from build123d import *

# Parameters (mm, degrees)
SKETCH1_W           = 39.99992
SKETCH1_H           = 19.99996
BOSS_EXTRUDE1_DEPTH = 3.499993
CUT_EXTRUDE1_START  = -2.00000108
CUT_EXTRUDE1_DEPTH  = 2.00000108


# Read off the part's stored shape, not the designer's step: Cut-Extrude1
with BuildPart() as part:
    # Sketch1 → Boss-Extrude1 (new body)
    with BuildSketch(Plane.XY):
        Rectangle(SKETCH1_W, SKETCH1_H)
    extrude(amount=BOSS_EXTRUDE1_DEPTH)

    # Sketch3 → section 0 of loft1
    with BuildSketch(Plane.XY.offset(5.99999308), mode=Mode.PRIVATE) as loft1_s0:
        with BuildLine():
            Line((-18.12500058, -8.375000014), (18.12500058, -8.375000014))
            Line((18.12500058, -8.375000014), (18.12500058, 8.375000014))
            Line((18.12500058, 8.375000014), (-18.12500058, 8.375000014))
            Line((-18.12500058, 8.375000014), (-18.12500058, -8.375000014))
        make_face()
    # loft up to a face of the part (loft1)
    loft([loft1_s0.sketch, part.faces().sort_by_distance((0, 0, 3.499993))[0]])

    # Cut-Extrude1 outline → Cut-Extrude1 (cut)
    with BuildSketch(Plane.XY.offset(5.99999308).offset(CUT_EXTRUDE1_START)):
        with BuildLine():
            ThreePointArc((-15.250002266, -8.375000014), (-16.092069776, -6.34206921), (-18.12500058, -5.5000017))
            Line((-18.12500058, -5.5000017), (-19.99996, -5.5000017))
            Line((-19.99996, -5.5000017), (-19.99996, -9.99998))
            Line((-19.99996, -9.99998), (-15.250002266, -9.99998))
            Line((-15.250002266, -9.99998), (-15.250002266, -8.375000014))
        make_face()
        with BuildLine():
            ThreePointArc((18.12500058, -5.5000017), (16.092069776, -6.34206921), (15.250002266, -8.375000014))
            Line((15.250002266, -8.375000014), (15.250002266, -9.99998))
            Line((15.250002266, -9.99998), (19.99996, -9.99998))
            Line((19.99996, -9.99998), (19.99996, -5.5000017))
            Line((19.99996, -5.5000017), (18.12500058, -5.5000017))
        make_face()
        with BuildLine():
            ThreePointArc((-18.12500058, 5.5000017), (-16.092069776, 6.34206921), (-15.250002266, 8.375000014))
            Line((-15.250002266, 8.375000014), (-15.250002266, 9.99998))
            Line((-15.250002266, 9.99998), (-19.99996, 9.99998))
            Line((-19.99996, 9.99998), (-19.99996, 5.5000017))
            Line((-19.99996, 5.5000017), (-18.12500058, 5.5000017))
        make_face()
        with BuildLine():
            ThreePointArc((15.250002266, 8.375000014), (16.092069776, 6.34206921), (18.12500058, 5.5000017))
            Line((18.12500058, 5.5000017), (19.99996, 5.5000017))
            Line((19.99996, 5.5000017), (19.99996, 9.99998))
            Line((19.99996, 9.99998), (15.250002266, 9.99998))
            Line((15.250002266, 9.99998), (15.250002266, 8.375000014))
        make_face()
    extrude(amount=CUT_EXTRUDE1_DEPTH, mode=Mode.SUBTRACT)


solid = part.part
Could you check a few things on this model? Use its own coordinates, in mm. A direction names the side the tool comes from. Give positions to 0.01 mm unless a question says otherwise; leave off trailing zeros. Answer as a JSON object with one key per item and string values.
Q1. Please list where these lines run through material, in increasing order: L1, parallel to X at y = -8.5, z = 4.3; L2, parallel to X at y = -1, z = 4.05; L3, parallel to Z at x = -18, y = 7.5.
Taken from the geometry:
{"L1": "x = -15.25 to 15.25", "L2": "x = -19.59 to 19.59", "L3": "z = 0 to 4"}
Q2. Will these pins go through, and if not, where does the flat tip stop? pin 1 Ø0.6 at (y, z) = (-8.5, 5) entering from -X; pin 2 Ø1.5 at (x, z) = (3, 5) entering from -Y; pin 3 Ø0.6 at (y, z) = (9, 5) entering from +X; pin 4 Ø0.7 at (x, z) = (-19, 5.5) entering from -Y.
Taken from the geometry:
{"pin 1": "stops at x = -15.26", "pin 2": "stops at y = -9.51", "pin 3": "stops at x = 15.25", "pin 4": "passes through"}
Q3. Which directions (+Z, -Z, +X, -X, +Y, -Y) give clear straight access to the entire face, cutting with the end or side of a thin tool? Please do faces 1 (the flat face through (-17, -8, 4)), 2 (the cylindrical face through (16.07, 6.365, 4.986)), 3 (the flat face through (17, -8, 4)).
Taken from the geometry:
{"face 1": "+Z, -X, -Y", "face 2": "+Z, +X, +Y", "face 3": "+Z, +X, -Y"}
